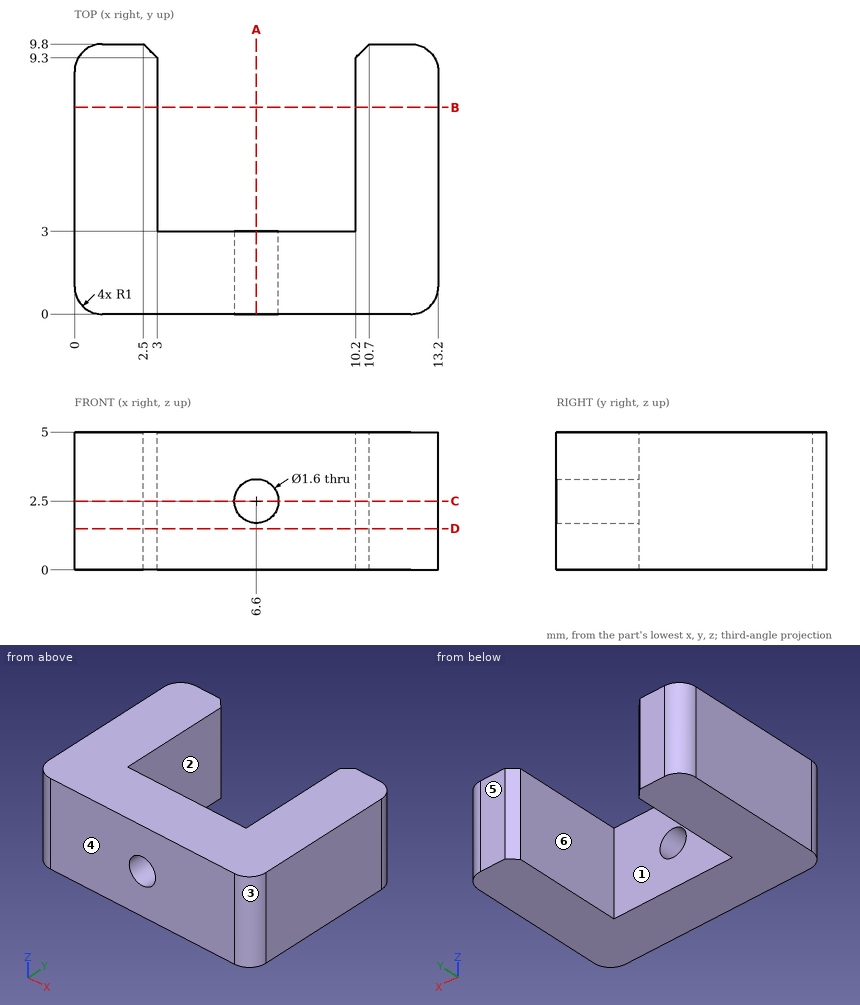
Input: dimensioned drawing with shaded views. Units: mm. Origin: part minimum x, y, z. A direction names the side the tool comes from. Give positions to 0.01 mm unless a question says otherwise; leave off trailing zeros. Write each loop counter-clockwise with the first axis right and the second up, starting at its lowest first coordinate (ties: lowest second). Pieces come first, ordered by that corner, then holes.
1. Section query A-A, the plane x = 6.6. Return loops of the section in (y, z).
2. Section query C-C, the plane z = 2.5. Return loops of the section in (x, y), then the cut area to 3 significant figures.
3. Pin query (flat end, axial travel): P1, Ø2, axis at y = 6, z = 2.5, coming from the -X side; P2, Ø1, axis at x = 9.5, z = 1.5, coming from the +Y side. Return the tip coordinate at first contact, or that it passes through.
4. Reachability of the marked faces 5 and 6 from +Z, -Z, +X, -X, +Y, -Y: full face, straight path, thin tool, end or side. Return the list, or none.
5. Line query: probe 1 along X at (y, z) = (3.75, 3.8); probe 2 along Z at (x, y) = (6.6, 2.35); probe 3 along Y at (x, z) = (8.25, 2.95). Output: solid intervals per line, ascending.
6. Draft query along X for the marked faces 1, 2, 3 and 4. Return one class per face: released by +X, released by -X, zero draft, split by the parting line, or undercut.
7. Section query D-D, the plane z = 1.5. Return loops of the section in (x, y).
8. Section query B-B, the plane y = 7.5. Return loops of the section in (x, z).
Computed:
1. outline: (0, 0) - (3, 0) - (3, 1.7) - (0, 1.7) - close; (0, 3.3) - (3, 3.3) - (3, 5) - (0, 5) - close
2. outline: (0, 1) arc R1 ccw to (1, 0) - (5.8, 0) - (5.8, 3) - (3, 3) - (3, 9.3) - (2.5, 9.8) - (1, 9.8) arc R1 ccw to (0, 8.8) - close; (7.4, 0) - (12.2, 0) arc R1 ccw to (13.2, 1) - (13.2, 8.8) arc R1 ccw to (12.2, 9.8) - (10.7, 9.8) - (10.2, 9.3) - (10.2, 3) - (7.4, 3) - close
2. area: 74.5 mm2
3. P1: stops at x = 0
3. P2: stops at y = 3
4. face 5: +Z, -Z, +X, -X, +Y
4. face 6: +Z, -Z, +Y
5. probe 1: x = 0 to 3, 10.2 to 13.2
5. probe 2: z = 0 to 1.7, 3.3 to 5
5. probe 3: y = 0 to 3
6. face 1: undercut
6. face 2: undercut
6. face 3: released by +X
6. face 4: zero draft
7. outline: (0, 1) arc R1 ccw to (1, 0) - (12.2, 0) arc R1 ccw to (13.2, 1) - (13.2, 8.8) arc R1 ccw to (12.2, 9.8) - (10.7, 9.8) - (10.2, 9.3) - (10.2, 3) - (3, 3) - (3, 9.3) - (2.5, 9.8) - (1, 9.8) arc R1 ccw to (0, 8.8) - close
8. outline: (0, 0) - (3, 0) - (3, 5) - (0, 5) - close; (10.2, 0) - (13.2, 0) - (13.2, 5) - (10.2, 5) - close
